```python
from build123d import *

# Parameters (mm, degrees)
SKETCH1_R           = 4
BOSS_EXTRUDE1_DEPTH = 6


with BuildPart() as part:
    # Sketch1 → Boss-Extrude1 (new body)
    with BuildSketch(Plane.XY):
        with BuildLine():
            Line((32.00713516, -18.923928181), (-10.976216134, -19.026159499))
            ThreePointArc((-10.976216134, -19.026159499), (-18.062653939, -16.105659467), (-21, -9.026187783))
            Line((-21, -9.026187783), (-21, 9.026187783))
            ThreePointArc((-21, 9.026187783), (-18.062653939, 16.105659467), (-10.976216134, 19.026159499))
            Line((-10.976216134, 19.026159499), (15.047567733, 18.964264704))
            ThreePointArc((15.047567733, 18.964264704), (29.158943369, 13.08962915), (35, -1.035678729))
            Line((35, -1.035678729), (35, -15.923936666))
            ThreePointArc((35, -15.923936666), (34.123841505, -18.042732848), (32.00713516, -18.923928181))
        make_face()
        with Locations((28, -12)):
            Circle(SKETCH1_R, mode=Mode.SUBTRACT)
        with BuildLine():
            Line((-10, 9.797958971), (-10, -9.797958971))
            ThreePointArc((-10, -9.797958971), (0, -14), (10, -9.797958971))
            Line((10, -9.797958971), (10, 9.797958971))
            ThreePointArc((10, 9.797958971), (0, 14), (-10, 9.797958971))
        make_face(mode=Mode.SUBTRACT)
    extrude(amount=BOSS_EXTRUDE1_DEPTH)


solid = part.part
```
Source: CAD feature listing. Evaluate the final solid. Frame: model axes, mm. A direction names the side the tool comes from. Give positions to 0.01 mm unless a question says otherwise; leave off trailing zeros. Loops run counter-clockwise (first coordinate to the right, second up) from the corner with the lowest first, then second, coordinate; pieces in that order, holes last. Notation, with made-up numbers: (49.25, 11.5) -> (58.25, 11.5) arc R18 cw to (58.25, 23.5) -> close; hole circle Ø10 at (-9, 67.5). An arc over 180 degrees is marked (long way). Put each result on its own line as item: value. Start each with the question number.
1) Reachability of faces 1 (the face through (14, 0, 0)), 2 (the face through (-10, 0, 3)) from +Z, -Z, +X, -X, +Y, -Y: full face, straight path, thin tool, end or side. Return the list, or none.
2) Contact query for a flat-ended pin moving along its axis: P1, Ø2, axis at x = 26.5, y = -13.5, coming from the +Z side. Output: stop coordinate, or through.
3) Draft query along X for faces 3 (the face through (34.147, -18.019, 2.958)), 4 (the face through (24.8, -14.4, 3)), 5 (the face through (-21, 0, 3)). Return one class per face: released by +X, released by -X, zero draft, split by the parting line, or undercut.
4) Material intervals for probe 1 along X at (y, z) = (-8.5, 2.85); probe 2 along X at (y, z) = (-4.5, 4.4); probe 3 along Y at (x, z) = (28, 3.7), sorted ascending.
5) Cut plane D-D (y = -12). Return loops of the section in (x, z), then the cut area to 3 significant figures.
6) Cut plane C-C (x = 28). Return loops of the section in (y, z), then the cut area to 3 significant figures.
7) Cut plane A-A (y = 6). Return loops of the section in (x, z), then the cut area to 3 significant figures.
8) Cut plane B-B (z = 1.25). Return loops of the section in (x, y).
Results are:
1. face 1: -Z, +X, -X, +Y, -Y
1. face 2: +Z, -Z
2. P1: passes through
3. face 3: released by +X
3. face 4: undercut
3. face 5: released by -X
4. probe 1: x = -21 to -10, 10 to 26.06, 29.94 to 35
4. probe 2: x = -21 to -10, 10 to 35
4. probe 3: y = -18.93 to -16, -8 to 14.16
5. outline: (-20.55, 0) -> (-7.21, 0) -> (-7.21, 6) -> (-20.55, 6) -> close; (7.21, 0) -> (24, 0) -> (24, 6) -> (7.21, 6) -> close; (32, 0) -> (35, 0) -> (35, 6) -> (32, 6) -> close
5. area: 199 mm2
6. outline: (-18.93, 0) -> (-16, 0) -> (-16, 6) -> (-18.93, 6) -> close; (-8, 0) -> (14.16, 0) -> (14.16, 6) -> (-8, 6) -> close
6. area: 151 mm2
7. outline: (-21, 0) -> (-10, 0) -> (-10, 6) -> (-21, 6) -> close; (10, 0) -> (33.72, 0) -> (33.72, 6) -> (10, 6) -> close
7. area: 208 mm2
8. outline: (-21, -9.03) arc R10 ccw to (-10.98, -19.03) -> (32.01, -18.92) arc R3 ccw to (35, -15.92) -> (35, -1.04) arc R20 ccw to (15.05, 18.96) -> (-10.98, 19.03) arc R10 ccw to (-21, 9.03) -> close; hole (-10, -9.8) arc R14 ccw to (10, -9.8) -> (10, 9.8) arc R14 ccw to (-10, 9.8) -> close; hole circle Ø8 at (28, -12)
